Read the model definition and answer for the solid it produces. Units are mm, in the model's axes. A direction names the side the tool comes from. Give positions to 0.01 mm unless a question says otherwise; leave off trailing zeros. Write each loop counter-clockwise with the first axis right and the second up, starting at its lowest first coordinate (ties: lowest second). Pieces come first, ordered by that corner, then holes. Notation, with made-up numbers: (62.25, -24) -> (92.25, -24) arc R24 ccw to (92.25, -14) -> close; hole circle Ø6 at (70, 17.25). An arc over 180 degrees is marked (long way). Answer as CSV lines item,"result". Start each with the question number.
1. The part is cut by section C-C, the plane x = -56.5. Determine the outline of the cut face in (y, z).
2. A tool of negligible diameter and unlimited length cuts with its end or side. For faces 5 (the flat face through (18.766, 39, 0)), 6 (the flat face through (35, 54, 4)), 7 (the flat face through (67, 7, -5)), 8 (the flat face through (-83.48, 5.58, 0.26)), 9 (the flat face through (-21, 5, 0)), from which of +Z, -Z, +X, -X, +Y, -Y can it reach the whole face along a straight path? Write none if from no direction.
3. The part is cut by section D-D, the plane x = 71.5. Determine the outline of the cut face in (y, z).
4. Given pin 1 (3.5 mm diameter, centred on y = 40, z = -2.5, fed in from -X); pin 2 (2 mm diameter, centred on y = 31, z = -12, fed in from -X); pin 3 (0.6 mm diameter, centred on y = 0.5, z = -0.5, fed in from +X), each flat-ended and moving along its own axis, determine where each tip first touches the part or whether it passes through.
5. Find the intervals of material crossed by line 1 (X direction, y = 42.5, z = 0); line 2 (X direction, y = 20.5, z = 0); line 3 (Z direction, x = 0, y = 19.25), in increasing order.
6. The part is cut by section A-A, the plane x = 31. Determine the outline of the cut face in (y, z).
7. The part is cut by section B-B, the plane y = 28.5. Determine the outline of the cut face in (x, z).
8. For a pull along Z with two mould halves and no side action, classify faces 1 (the flat face through (-1, 15, 18.5)), 2 (the flat face through (60, 11, 4)), 3 (the cylindrical face through (-36, 31, 0)), 4 (the cylindrical face through (-3, 19, 0)) as pulls with the +Z half, pulls with the -Z half, needs draft (parallel to the pull), parting line crosses it, or undercut.
from build123d import *

# Parameters (mm, degrees)
BOSS_EXTRUDE1_DEPTH = 18.5
BOSS_EXTRUDE2_START = -11
BOSS_EXTRUDE2_DEPTH = 54
CUT_EXTRUDE1_DEPTH  = 27
SKETCH4_R           = 5
CUT_EXTRUDE2_DEPTH  = 55
SKETCH5_W           = 20
SKETCH5_H           = 20
CUT_EXTRUDE3_DEPTH  = 8
SKETCH6_W           = 71
SKETCH6_H           = 2
CUT_EXTRUDE4_DEPTH  = 11
CUT_EXTRUDE5_DEPTH  = 12
FILLET1_R           = 6


with BuildPart() as part:
    # Sketch1 → Boss-Extrude1 (new body, symmetric)
    with BuildSketch(Plane.XY):
        Polygon((-85, 0), (85, 0), (82, 11), (-82, 11), align=None)
    extrude(amount=BOSS_EXTRUDE1_DEPTH, both=True)

    # Sketch2 → Boss-Extrude2 (add)
    with BuildSketch(Plane(origin=(0, 11, 0), x_dir=(1, 0, 0), z_dir=(0, 1, 0)).offset(BOSS_EXTRUDE2_START)):
        with BuildLine():
            Line((38.816877772, -18.5), (-38.816877772, -18.5))
            ThreePointArc((-38.816877772, -18.5), (-43, 0), (-38.816877772, 18.5))
            Line((-38.816877772, 18.5), (38.816877772, 18.5))
            ThreePointArc((38.816877772, 18.5), (43, 0), (38.816877772, -18.5))
        make_face()
    extrude(amount=BOSS_EXTRUDE2_DEPTH)

    # Sketch3 → Cut-Extrude1 (cut, symmetric)
    with BuildSketch(Plane.XY):
        with BuildLine():
            Line((-22, 54), (-22, 41))
            Line((-22, 41), (-18.766334066, 41))
            Line((-18.766334066, 41), (-18.766334066, 38))
            ThreePointArc((-18.766334066, 38), (0, 21.970640627), (18.766334066, 38))
            Line((18.766334066, 38), (18.766334066, 41))
            Line((18.766334066, 41), (22, 41))
            Line((22, 41), (22, 54))
            Line((22, 54), (-22, 54))
        make_face()
    extrude(amount=CUT_EXTRUDE1_DEPTH, both=True, mode=Mode.SUBTRACT)

    # Sketch4 → Cut-Extrude2 (cut, through all)
    with BuildSketch(Plane(origin=(0, 54, 0), x_dir=(1, 0, 0), z_dir=(0, 1, 0))):
        with Locations((-31, 0)):
            Circle(SKETCH4_R)
        with Locations((31, 0)):
            Circle(SKETCH4_R)
    extrude(amount=-CUT_EXTRUDE2_DEPTH, mode=Mode.SUBTRACT)

    # Sketch5 → Cut-Extrude3 (cut)
    with BuildSketch(Plane.XZ):
        with Locations((-31, 0)):
            Rectangle(SKETCH5_W, SKETCH5_H)
        with Locations((31, 0)):
            Rectangle(SKETCH5_W, SKETCH5_H)
    extrude(amount=-CUT_EXTRUDE3_DEPTH, mode=Mode.SUBTRACT)

    # Sketch6 → Cut-Extrude4 (cut, symmetric)
    with BuildSketch(Plane.XY):
        with Locations((-39.5, 1)):
            Rectangle(SKETCH6_W, SKETCH6_H)
    cut_extrude4 = extrude(amount=CUT_EXTRUDE4_DEPTH, both=True, mode=Mode.SUBTRACT)

    # Mirror1: Cut-Extrude4 across plane
    add(cut_extrude4.mirror(Plane(origin=(0, 0, 0), x_dir=(0, 0, 1), z_dir=(1, 0, 0))), mode=Mode.SUBTRACT)

    # Sketch7 → Cut-Extrude5 (cut, through all)
    with BuildSketch(Plane(origin=(0, 11, 0), x_dir=(1, 0, 0), z_dir=(0, 1, 0))):
        with BuildLine():
            Line((-64, -5), (-70, -5))
            ThreePointArc((-70, -5), (-75, 0), (-70, 5))
            Line((-70, 5), (-64, 5))
            ThreePointArc((-64, 5), (-59, 0), (-64, -5))
        make_face()
        with BuildLine():
            Line((64, -5), (70, -5))
            ThreePointArc((70, -5), (75, 0), (70, 5))
            Line((70, 5), (64, 5))
            ThreePointArc((64, 5), (59, 0), (64, -5))
        make_face()
    extrude(amount=-CUT_EXTRUDE5_DEPTH, mode=Mode.SUBTRACT)

    # Sketch8 → Cut-Revolve1 (revolve, cut)
    with BuildSketch(Plane.XY):
        Polygon((0, 21.970640627), (0, 14.16805877), (3, 15.970640627), (3, 25.476225131), (0, 25.476225131), align=None)
    revolve(axis=Axis((0, 21.970640627, 0), (0, -1, 0)), mode=Mode.SUBTRACT)

    # Fillet1
    fillet1_edges = [part.edges().sort_by_distance(p)[0] for p in [
        (-43, 11, 0),
        (43, 11, 0),
    ]]
    fillet(fillet1_edges, radius=FILLET1_R)


solid = part.part
Results found:
1,outline,"(0, -18.5) -> (11, -18.5) -> (11, 18.5) -> (0, 18.5) -> (0, 11) -> (2, 11) -> (2, -11) -> (0, -11) -> close"
2,face 5,"+Z, -Z, +Y"
2,face 6,"+Z, -Z, +X, -X, +Y"
2,face 7,"+Y, -Y"
2,face 8,"+Z, -Z, -X, +Y"
2,face 9,"-Y"
3,outline,"(0, -18.5) -> (11, -18.5) -> (11, -4.77) -> (2, -4.77) -> (2, -11) -> (0, -11) -> close; (0, 11) -> (2, 11) -> (2, 4.77) -> (11, 4.77) -> (11, 18.5) -> (0, 18.5) -> close"
4,pin 1,"stops at x = -42.99"
4,pin 2,"stops at x = -41.57"
4,pin 3,"stops at x = 84.95"
5,line 1,"x = -43 to -36, -26 to -22, 22 to 26, 36 to 43"
5,line 2,"x = -43 to -36, -26 to -3, 3 to 26, 36 to 43"
5,line 3,"z = -18.5 to -3, 3 to 18.5"
6,outline,"(0, -18.5) -> (54, -18.5) -> (54, -5) -> (8, -5) -> (8, -10) -> (2, -10) -> (2, -11) -> (0, -11) -> close; (0, 11) -> (2, 11) -> (2, 10) -> (8, 10) -> (8, 5) -> (54, 5) -> (54, 18.5) -> (0, 18.5) -> close"
7,outline,"(-38.82, -18.5) -> (-14.33, -18.5) -> (-14.33, 18.5) -> (-38.82, 18.5) arc R43 ccw to start; (14.33, -18.5) -> (38.82, -18.5) arc R43 ccw to (38.82, 18.5) -> (14.33, 18.5) -> close; hole circle Ø10 at (-31, 0); hole circle Ø10 at (31, 0)"
8,face 1,"pulls with the +Z half"
8,face 2,"needs draft"
8,face 3,"undercut"
8,face 4,"undercut"
